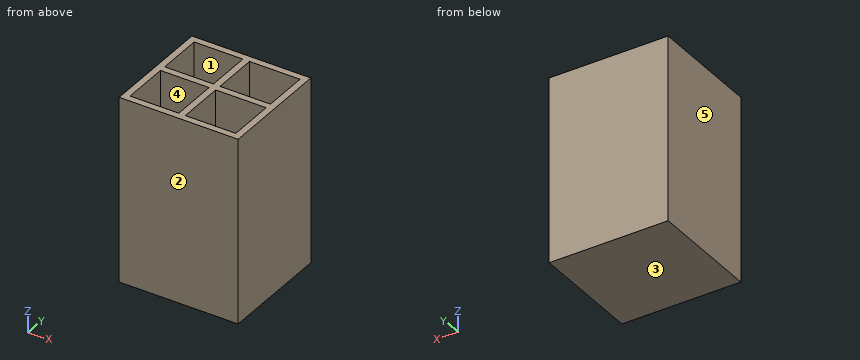
```python
from build123d import *

# Parameters (mm, degrees)
F0_W      = 57.15
F0_H      = 88.9
F1_DEPTH  = 3.175
F2_W      = 3.175
F2_H      = 88.9
F3_DEPTH  = 50.8
F4_W      = 3.175
F4_H      = 88.9
F5_DEPTH  = 50.8
F6_W      = 53.0491641998
F6_H      = 88.9
F7_DEPTH  = 3.175
F8_W      = 50.8
F8_H      = 47.625
F9_DEPTH  = 3.175
F11_W     = 50.8
F11_H     = 47.625
F12_DEPTH = 3.175
F13_W     = 3.175
F13_H     = 85.725
F14_DEPTH = 50.8
F15_W     = 3.175
F15_H     = 85.725
F16_DEPTH = 50.8


with BuildPart() as f1:
    # F0 (on Front) → F1 (new body)
    with BuildSketch(Plane.XZ):
        with Locations((6.8577993661, 8.5990129304)):
            Rectangle(F0_W, F0_H)
    extrude(amount=F1_DEPTH)

    # F2 (on face) → F3 (join)
    with BuildSketch(Plane.XZ.offset(3.175)):
        with Locations((-20.1297006339, 8.5990129304)):
            Rectangle(F2_W, F2_H)
    extrude(amount=F3_DEPTH)

    # F4 (on face) → F5 (join)
    with BuildSketch(Plane.XZ.offset(3.175)):
        with Locations((33.8452993661, 8.5990129304)):
            Rectangle(F4_W, F4_H)
    extrude(amount=F5_DEPTH)

    # F6 (on face) → F7 (join)
    with BuildSketch(Plane.XZ.offset(53.975)):
        with Locations((5.7332172662, 8.5990129304)):
            Rectangle(F6_W, F6_H)
    extrude(amount=-F7_DEPTH)

    # F11 (on face) → F12 (join)
    with BuildSketch(Plane(origin=(0, 0, -35.8509870696), x_dir=(1, 0, 0), z_dir=(0, 0, -1))):
        with Locations((6.8577993661, 26.9875)):
            Rectangle(F11_W, F11_H)
    extrude(amount=-F12_DEPTH)

    # F13 (on face) → F14 (join)
    with BuildSketch(Plane.XZ.offset(3.175)):
        with Locations((6.430921746, 10.1865129304)):
            Rectangle(F13_W, F13_H)
    extrude(amount=F14_DEPTH)

    # F15 (on face) → F16 (join)
    with BuildSketch(Plane.YZ.offset(-18.5422006339)):
        with Locations((-26.6523276031, 10.1865129304)):
            Rectangle(F15_W, F15_H)
    extrude(amount=F16_DEPTH)


with BuildPart() as f9:
    # F8 (on face) → F9 (new body)
    with BuildSketch(Plane(origin=(0, 0, -35.8509870696), x_dir=(1, 0, 0), z_dir=(0, 0, -1))):
        with Locations((6.8577993661, 26.9875)):
            Rectangle(F8_W, F8_H)
    extrude(amount=-F9_DEPTH)


solid = f1.part
```
CAD build for the part. Positions are in the model's coordinates, mm. Face numbers are marked on the shaded views. A direction names the side the tool comes from. Give positions to 0.01 mm unless a question says otherwise; leave off trailing zeros. Order: outer loops, then holes, each group sorted by start corner. A loop starts at its lowest first (then second) coordinate and runs counter-clockwise, first axis right, second up.
(1) Drill centre lines: L1, parallel to X at y = -50, z = 47; L2, parallel to Y at x = -2, z = 44 (3 decimals); L3, parallel to Z at x = -9.5, y = -14. Where is each one in solid material? Low to high.
(2) Tool access for the marked faces 4 and 5: list every direction of +Z, -Z, +X, -X, +Y, -Y with a clear straight run to the whole face (end or side of a thin tool).
(3) Saw through at C-C, the plane y = -5. Give the cut face in (x, z).
(4) Flat gauge pins, fed straight in: pin 1 (6.5 mm diameter, centred on x = 22.5, y = -10, fed in from +Z); pin 2 (24 mm diameter, centred on x = -9.5, y = -16, fed in from +Z). Where does each tip first touch, or does it go through?
(5) Saw through at A-A, the plane z = -22. Give the cut face in (x, y) (3 decimals).
(6) Mould opens along Y. For the marked faces 1, 2 and 3 say: released by +Y, released by -Y, zero draft, split by the parting line, or undercut.
(7) Saw through at B-B, the plane x = 28. Give the cut face in (y, z) (3 decimals), then the cut area to 3 significant figures.
Results found:
1. L1: x = -21.72 to -18.54, 4.84 to 8.02, 32.26 to 35.43
1. L2: y = -53.975 to -50.8, -28.24 to -25.065, -3.175 to 0
1. L3: z = -35.85 to -32.68
2. face 4: +Z
2. face 5: +Z, -Z, -X, +Y, -Y
3. outline: (-21.72, -35.85) - (35.43, -35.85) - (35.43, 53.05) - (32.26, 53.05) - (32.26, -32.68) - (8.02, -32.68) - (8.02, 53.05) - (4.84, 53.05) - (4.84, -32.68) - (-18.54, -32.68) - (-18.54, 53.05) - (-21.72, 53.05) - close
4. pin 1: stops at z = -32.68
4. pin 2: stops at z = 53.05
5. outline: (-21.717, -53.975) - (35.433, -53.975) - (35.433, 0) - (-21.717, 0) - close; hole (-18.542, -50.8) - (4.843, -50.8) - (4.843, -28.24) - (-18.542, -28.24) - close; hole (-18.542, -25.065) - (4.843, -25.065) - (4.843, -3.175) - (-18.542, -3.175) - close; hole (8.018, -50.8) - (32.258, -50.8) - (32.258, -28.24) - (8.018, -28.24) - close; hole (8.018, -25.065) - (32.258, -25.065) - (32.258, -3.175) - (8.018, -3.175) - close
6. face 1: undercut
6. face 2: released by -Y
6. face 3: zero draft
7. outline: (-53.975, -35.851) - (0, -35.851) - (0, 53.049) - (-3.175, 53.049) - (-3.175, -32.676) - (-25.065, -32.676) - (-25.065, 53.049) - (-28.24, 53.049) - (-28.24, -32.676) - (-50.8, -32.676) - (-50.8, 53.049) - (-53.975, 53.049) - close
7. area: 988 mm2
